Here's how the part is built. I have some questions about the finished solid (model axes, mm). A direction names the side the tool comes from. Give positions to 0.01 mm unless a question says otherwise; leave off trailing zeros. Loops run counter-clockwise (first coordinate to the right, second up) from the corner with the lowest first, then second, coordinate; pieces in that order, holes last. Notation, with made-up numbers: (41.25, 47) - (73.25, 47) arc R31 cw to (73.25, 76) - close; hole circle Ø6 at (68.25, 3). An arc over 180 degrees is marked (long way). Use a Markdown table: item, result.
from build123d import *

# Parameters (mm, degrees)
SKETCH1_W           = 162
SKETCH1_H           = 232
BOSS_EXTRUDE1_DEPTH = 4
SKETCH4_W           = 30
SKETCH4_H           = 21
SKETCH4_W_2         = 21
CUT_EXTRUDE3_DEPTH  = 148.108803272
SKETCH5_R           = 1.599999999
SKETCH5_R_2         = 1.600000001
SKETCH5_R_3         = 1.6
SKETCH5_R_4         = 2
CUT_EXTRUDE4_DEPTH  = 148.108803272
SKETCH7_W           = 65
SKETCH7_H           = 75
CUT_EXTRUDE6_DEPTH  = 148.108803272
CUT_EXTRUDE7_DEPTH  = 148.108803272
CUT_EXTRUDE8_DEPTH  = 148.108803272
SKETCH10_R          = 2.5
CUT_EXTRUDE9_DEPTH  = 148.108803272
CUT_EXTRUDE10_DEPTH = 4
SKETCH12_W          = 12
SKETCH12_H          = 70
CUT_EXTRUDE11_DEPTH = 4


with BuildPart() as part:
    # Sketch1 → Boss-Extrude1 (new body)
    with BuildSketch(Plane(origin=(0, 0, 0), x_dir=(1, 0, 0), z_dir=(0, 1, 0))):
        with Locations((4, 4)):
            Rectangle(SKETCH1_W, SKETCH1_H)
    extrude(amount=BOSS_EXTRUDE1_DEPTH)

    # Sketch4 → Cut-Extrude3 (cut, through all)
    with BuildSketch(Plane(origin=(0, 4, 0), x_dir=(1, 0, 0), z_dir=(0, 1, 0))):
        with Locations((70, 109.5)):
            Rectangle(SKETCH4_W, SKETCH4_H)
        with Locations((-66.5, 4)):
            Rectangle(SKETCH4_W_2, SKETCH4_H)
        with Locations((70, -101.5)):
            Rectangle(SKETCH4_W, SKETCH4_H)
    extrude(amount=-CUT_EXTRUDE3_DEPTH, mode=Mode.SUBTRACT)

    # Sketch5 → Cut-Extrude4 (cut, through all)
    with BuildSketch(Plane.XZ):
        with Locations(Location((-48.000025976, -4, 0), (0, 0, 270))):
            Circle(SKETCH5_R)
        with Locations(Location((46.999999998, -109.999999999, 0), (0, 0, 270))):
            Circle(SKETCH5_R_2)
        with Locations(Location((46.999999999, 101.999999999, 0), (0, 0, 270))):
            Circle(SKETCH5_R_3)
        with Locations(Location((41.3, 37.25, 0), (0, 0, 270))):
            Circle(SKETCH5_R_4)
        with Locations(Location((41.3, 77.25, 0), (0, 0, 270))):
            Circle(SKETCH5_R_4)
        with Locations(Location((1.3, 37.25, 0), (0, 0, 270))):
            Circle(SKETCH5_R_4)
        with Locations(Location((1.3, 77.25, 0), (0, 0, 270))):
            Circle(SKETCH5_R_4)
        with Locations(Location((41.3, -45.25, 0), (0, 0, 270))):
            Circle(SKETCH5_R_4)
        with Locations(Location((1.3, -45.25, 0), (0, 0, 270))):
            Circle(SKETCH5_R_4)
        with Locations(Location((1.3, -85.25, 0), (0, 0, 270))):
            Circle(SKETCH5_R_4)
        with Locations(Location((41.3, -85.25, 0), (0, 0, 270))):
            Circle(SKETCH5_R_4)
    extrude(amount=-CUT_EXTRUDE4_DEPTH, mode=Mode.SUBTRACT)

    # Sketch7 → Cut-Extrude6 (cut, through all)
    with BuildSketch(Plane.XZ):
        with Locations((-44.5, -82.5)):
            Rectangle(SKETCH7_W, SKETCH7_H)
    extrude(amount=-CUT_EXTRUDE6_DEPTH, mode=Mode.SUBTRACT)

    # Sketch8 → Cut-Extrude7 (cut, through all)
    with BuildSketch(Plane.XZ):
        with BuildLine():
            Line((-47, 92), (-37, 92))
            ThreePointArc((-37, 92), (-29.928932188, 89.071067812), (-27, 82))
            Line((-27, 82), (-27, 32))
            ThreePointArc((-27, 32), (-29.928932188, 24.928932188), (-37, 22))
            Line((-37, 22), (-47, 22))
            ThreePointArc((-47, 22), (-54.071067812, 24.928932188), (-57, 32))
            Line((-57, 32), (-57, 82))
            ThreePointArc((-57, 82), (-54.071067812, 89.071067812), (-47, 92))
        make_face()
    extrude(amount=-CUT_EXTRUDE7_DEPTH, mode=Mode.SUBTRACT)

    # Sketch9 → Cut-Extrude8 (cut, through all)
    with BuildSketch(Plane(origin=(0, 4, 0), x_dir=(1, 0, 0), z_dir=(0, 1, 0))):
        with BuildLine():
            Line((28, 100), (32, 100))
            ThreePointArc((32, 100), (34.121320344, 100.878679656), (35, 103))
            Line((35, 103), (35, 107))
            ThreePointArc((35, 107), (34.121320344, 109.121320344), (32, 110))
            Line((32, 110), (28, 110))
            ThreePointArc((28, 110), (25.878679656, 109.121320344), (25, 107))
            Line((25, 107), (25, 103))
            ThreePointArc((25, 103), (25.878679656, 100.878679656), (28, 100))
        make_face()
    extrude(amount=-CUT_EXTRUDE8_DEPTH, mode=Mode.SUBTRACT)

    # Sketch10 → Cut-Extrude9 (cut, through all)
    with BuildSketch(Plane(origin=(0, 4, 0), x_dir=(1, 0, 0), z_dir=(0, 1, 0))):
        with Locations(Location((12, -11.291947097, 0), (0, 0, 270))):
            Circle(SKETCH10_R)
        with Locations(Location((12, 4.708052903, 0), (0, 0, 270))):
            Circle(SKETCH10_R)
        with Locations(Location((77, 4.708052903, 0), (0, 0, 270))):
            Circle(SKETCH10_R)
        with Locations(Location((77, -11.291947097, 0), (0, 0, 270))):
            Circle(SKETCH10_R)
    extrude(amount=-CUT_EXTRUDE9_DEPTH, mode=Mode.SUBTRACT)

    # Sketch11 → Cut-Extrude10 (cut)
    with BuildSketch(Plane(origin=(0, 4, 0), x_dir=(1, 0, 0), z_dir=(0, 1, 0))):
        with BuildLine():
            Line((-36, 6), (-6, 6))
            ThreePointArc((-6, 6), (-4, 4), (-6, 2))
            Line((-6, 2), (-36, 2))
            ThreePointArc((-36, 2), (-38, 4), (-36, 6))
        make_face()
    extrude(amount=-CUT_EXTRUDE10_DEPTH, mode=Mode.SUBTRACT)

    # Sketch12 → Cut-Extrude11 (cut)
    with BuildSketch(Plane(origin=(0, 4, 0), x_dir=(1, 0, 0), z_dir=(0, 1, 0))):
        with Locations((79, 64)):
            Rectangle(SKETCH12_W, SKETCH12_H)
        with Locations((79, -56)):
            Rectangle(SKETCH12_W, SKETCH12_H)
    extrude(amount=-CUT_EXTRUDE11_DEPTH, mode=Mode.SUBTRACT)


solid = part.part
(1) Suppose I cut it at A-A on z = 43.5. Write out the boundary of the cut face in (x, y).
A:
| item | result |
|---|---|
| outline | (-77, 0) - (-57, 0) - (-57, 4) - (-77, 4) - close; (-27, 0) - (73, 0) - (73, 4) - (-27, 4) - close |
(2) Suppose I cut it at C-C on z = -31.5. Write out the boundary of the cut face in (x, y), plus the area to 3 significant figures.
A:
| item | result |
|---|---|
| outline | (-77, 0) - (73, 0) - (73, 4) - (-77, 4) - close |
| area | 600 mm2 |
(3) On a 3-axis mill with a long thin cutter (end or side, diameter ignored), from which of +Z, -Z, +X, -X, +Y, -Y can I reach the whole of each face in a straight line? I mean faces 3 (the face through (-29.85, 1.97, 25.01)), 4 (the face through (3, 4, 20)). Say none if no direction works.
A:
| item | result |
|---|---|
| face 3 | +Y, -Y |
| face 4 | +Z, -Z, +X, -X, +Y |
(4) Will these pins go through, and if not, where does the flat tip stop? pin 1 (3 mm diameter, centred on x = 41.3, z = -85.25, fed in from -Y); pin 2 (1.5 mm diameter, centred on y = 1.5, z = -94.5, fed in from -X); pin 3 (1.2 mm diameter, centred on y = 1.5, z = 106, fed in from +X); pin 4 (1 mm diameter, centred on y = 0.5, z = 61.5, fed in from +X).
A:
| item | result |
|---|---|
| pin 1 | through |
| pin 2 | x = -12 |
| pin 3 | x = 55 |
| pin 4 | x = 73 |
(5) We'd pull the mould along Z, two halves only. Please class faces 1 (the face through (3, 0, 20)), 2 (the face through (9.56, 2.03, -5.25)): pulls with the +Z half, pulls with the -Z half, needs draft (parallel to the pull), parting line crosses it, or undercut.
A:
| item | result |
|---|---|
| face 1 | needs draft |
| face 2 | undercut |
(6) Suppose I cut it at B-B on y = 2.95. Count the separate pieces of the cut face and the enclosed holes in it, plus the area to 3 significant figures.
A:
| item | result |
|---|---|
| separate pieces | 1 |
| enclosed holes | 18 |
| area | 26,900 mm2 |
(7) If I drill on line 1 (Z direction, x = 47, y = 1.95); line 2 (X direction, y = 3.15, z = -45.25); line 3 (X direction, y = 2.1, z = 37.25), over which ranges is the centre line in solid material (lowest first)?
A:
| item | result |
|---|---|
| line 1 | -120 to -111.6, -108.4 to 100.4, 103.6 to 112 |
| line 2 | -12 to -0.7, 3.3 to 39.3, 43.3 to 73 |
| line 3 | -77 to -57, -27 to -0.7, 3.3 to 39.3, 43.3 to 73 |
